```python
from build123d import *

# Parameters (mm, degrees)
F0_R     = 4.9836691613
F0_W     = 15.3446597978
F0_H     = 18.0084193125
F0_W_2   = 14.8993115872
F1_DEPTH = 12.7
F2_DEPTH = 50.8
F3_R     = 5.08
F6_D     = 6.35
F5_W     = 18.0084193125
F5_H     = 9.8407220423
F7_DEPTH = 17.78
F9_DEPTH = 25.4


with BuildPart() as f1:
    # F0 (on Top) → F1 (new body)
    with BuildSketch(Plane.XY):
        with BuildLine():
            Line((36.0745033145, 16.2670928985), (-40.1254966855, 16.2670928985))
            ThreePointArc((-40.1254966855, 16.2670928985), (-52.1476034559, -1.2861349798), (-38.2574259843, -17.4016501734))
            Line((-38.2574259843, -17.4016501734), (37.9416596259, -17.0283511457))
            ThreePointArc((37.9416596259, -17.0283511457), (49.3126119569, 0.3093896587), (36.0745033145, 16.2670928985))
        make_face()
        with Locations((31.8983709386, -0.6671736808)):
            Circle(F0_R, mode=Mode.SUBTRACT)
        with Locations((-34.7327866279, -0.3198943033)):
            Circle(F0_R, mode=Mode.SUBTRACT)
        with Locations((-17.6295996644, -0.2460409887)):
            Rectangle(F0_W, F0_H, mode=Mode.SUBTRACT)
        with Locations((15.2155896649, -0.2460409887)):
            Rectangle(F0_W_2, F0_H, mode=Mode.SUBTRACT)
        with Locations((-17.6295996644, -0.2460409887)):
            Rectangle(F0_W, F0_H)
        with Locations((15.2155896649, -0.2460409887)):
            Rectangle(F0_W_2, F0_H)
    extrude(amount=F1_DEPTH)

    # F0 (on Top) → F2 (join)
    with BuildSketch(Plane.XY):
        with Locations((-17.6295996644, -0.2460409887)):
            Rectangle(F0_W, F0_H)
        with Locations((15.2155896649, -0.2460409887)):
            Rectangle(F0_W_2, F0_H)
    extrude(amount=F2_DEPTH)

    # F3
    f3_edges = [f1.edges().sort_by_distance(p)[0] for p in [
        (-17.6296, -9.250251, 50.8),
        (-17.6296, 8.758169, 50.8),
        (15.21559, 8.758169, 50.8),
        (15.21559, -9.250251, 50.8),
    ]]
    fillet(f3_edges, radius=F3_R)

    # F6 (through all)
    with Locations(Plane(origin=(-25.3019295633, 0, 0), x_dir=(0, -1, 0), z_dir=(-1, 0, 0))):
        with Locations((0, 43.0034697056)):
            Hole(F6_D / 2)

    # F5 (on face) → F7 (join)
    with BuildSketch(Plane.YZ.offset(-9.9572697654)):
        with Locations((-0.2460409887, 17.6203610212)):
            Rectangle(F5_W, F5_H)
    extrude(amount=F7_DEPTH)

    # F8 (on face) → F9 (cut)
    with BuildSketch(Plane.XZ.offset(9.250250645)):
        with BuildLine():
            Line((7.7659338713, 22.5407220423), (-9.9572697654, 22.5407220423))
            ThreePointArc((-9.9572697654, 22.5407220423), (-1.0956679471, 16.072257104), (7.7659338713, 22.5407220423))
        make_face()
    extrude(amount=-F9_DEPTH, mode=Mode.SUBTRACT)


solid = f1.part
```
For this review, take the finished solid that the model builds, in its own axes (mm). A direction names the side the tool comes from. Coordinates: 2 decimals unless noted, no trailing zeros. Order: outer loops, then holes, each group sorted by start corner. A loop starts at its lowest first (then second) coordinate and runs counter-clockwise, first axis right, second up. Notation, with made-up numbers: (61, 54.25) - (114, 54.25) arc R13 ccw to (114, 69.25) - close; hole circle Ø8 at (62.5, 85.5). An arc over 180 degrees is marked (long way). Answer as a JSON object with one key per item and string values. Group by question number.
1. We need section B-B on z = 44. State the section outline as (x, y) points.
2. Clearance check with flat-ended pins moving along their axes: P1, Ø10, axis at y = 4, z = 16.5, coming from the -X side; P2, Ø11.5, axis at x = -34.73, y = -0.32, coming from the -Z side; P3, Ø14.5, axis at y = -4, z = 35.5, coming from the -X side; P4, Ø9, axis at y = -1, z = 25, coming from the +X side. State where each tip first meets the part, or that it passes through.
3. For faces 1 (the flat face through (-2, 11, 12.7)), 2 (the flat face through (-12, -9.25, 29)), 3 (the flat face through (-25.302, 0, 31)), 4 (the flat face through (-9.957, 0, 36)), list the 3-axis set-ups (+Z, -Z, +X, -X, +Y, -Y) from which the entire face can be reached by the end or side of a thin tool; tool diameter is ignored.
4. The part is to be moulded in two halves that separate along Y. For faces 5 (the cylindrical face through (-30.13, -2.23, 6.26)), 6 (the cylindrical face through (15.32, 7.31, 49.27)), 7 (the flat face through (22.665, 0, 31)), say which applies: pulls with the +Y half, pulls with the -Y half, needs draft (parallel to the pull), parting line crosses it, or undercut.
5. We need section D-D on x = 42. State the section outline as (y, z) points, then the cut area to 3 significant figures.
6. We need section C-C on y = 6. State the section outline as (x, z) points.
7. We need section A-A on z = 26.5. State the section outline as (x, y) points.
8. For probe 1 along Z at (x, y) = (-20, 0); probe 2 along X at (y, z) = (-4.5, 47.5); probe 3 along Z at (x, y) = (36.5, 11), list the stretches that pass through material, from the lowest coordinate up.
Final values:
{
 "1": {"outline": "(-25.3, -9.25) - (-9.96, -9.25) - (-9.96, -3.01) - (-25.3, -3.01) - close; (-25.3, 3.01) - (-9.96, 3.01) - (-9.96, 8.76) - (-25.3, 8.76) - close; (7.77, -9.25) - (22.67, -9.25) - (22.67, -3.01) - (7.77, -3.01) - close; (7.77, 3.01) - (22.67, 3.01) - (22.67, 8.76) - (7.77, 8.76) - close"},
 "2": {"P1": "x = -52.14", "P2": "z = 0", "P3": "x = -25.3", "P4": "x = 22.67"},
 "3": {"face 1": "+Z", "face 2": "+Z, +X, -X, -Y", "face 3": "+Z, -X, +Y, -Y", "face 4": "+Z, +Y, -Y"},
 "4": {"face 5": "undercut", "face 6": "pulls with the +Y half", "face 7": "needs draft"},
 "5": {"outline": "(-14.89, 0) - (13.55, 0) - (13.55, 12.7) - (-14.89, 12.7) - close", "area": "361 mm²"},
 "6": {"outline": "(-50.99, 0) - (48.02, 0) - (48.02, 12.7) - (22.67, 12.7) - (22.67, 50.24) - (7.77, 50.24) - (7.77, 22.54) arc R9.3 cw to (-9.96, 22.54) - (-9.96, 50.24) - (-25.3, 50.24) - (-25.3, 12.7) - (-50.99, 12.7) - close"},
 "7": {"outline": "(-25.3, -9.25) - (-9.96, -9.25) - (-9.96, 8.76) - (-25.3, 8.76) - close; (7.77, -9.25) - (22.67, -9.25) - (22.67, 8.76) - (7.77, 8.76) - close"},
 "8": {"probe 1": "0 to 39.83, 46.18 to 50.8", "probe 2": "-25.3 to -9.96, 7.77 to 22.67", "probe 3": "0 to 12.7"}
}
